Here's how the part is built. I have some questions about the finished solid (model axes, mm). A direction names the side the tool comes from. Coordinates: 2 decimals unless noted, no trailing zeros. Write each loop counter-clockwise with the first axis right and the second up, starting at its lowest first coordinate (ties: lowest second). Pieces come first, ordered by that corner, then holes.
```python
from build123d import *

# Parameters (mm, degrees)
EXTRUDE1_DEPTH      = 3
EXTRUDE1_DEPTH_BACK = 3
SKETCH2_OUTSIDE_W   = 52.392
SKETCH2_OUTSIDE_H   = 53.94
SKETCH2_OUTSIDE_R   = 5
CUT_EXTRUDE1_DEPTH  = 10.712534856
CUT_EXTRUDE1_DRAFT  = 60
SKETCH3_OUTSIDE_W   = 52.392
SKETCH3_OUTSIDE_H   = 53.94
SKETCH3_OUTSIDE_R   = 5
CUT_EXTRUDE2_DEPTH  = 10.712534856
CUT_EXTRUDE2_DRAFT  = 60
SKETCH4_R           = 3
CUT_EXTRUDE3_DEPTH  = 10.712534856
CUT_EXTRUDE7_DEPTH  = 0.635


with BuildPart() as part:
    # Sketch1 → Extrude1 (new, two sides: drawn at the far end of the back side and taken through both)
    with BuildSketch(Plane.XY.offset(-EXTRUDE1_DEPTH_BACK)):
        Polygon((0, 5.773502692), (-5, 2.886751346), (-5, -2.886751346), (0, -5.773502692), (5, -2.886751346), (5, 2.886751346), align=None)
    extrude(amount=EXTRUDE1_DEPTH + EXTRUDE1_DEPTH_BACK)


with BuildPart() as cut_extrude1_tool:
    # Sketch2 outside → Cut-Extrude1 (with draft: the straight prism first)
    with BuildSketch(Plane(origin=(0, 0, 3), x_dir=(-1, 0, 0), z_dir=(0, 0, -1))):
        Rectangle(SKETCH2_OUTSIDE_W, SKETCH2_OUTSIDE_H)
        Circle(SKETCH2_OUTSIDE_R, mode=Mode.SUBTRACT)
    extrude(amount=CUT_EXTRUDE1_DEPTH)
    # Cut-Extrude1: the draft: its side faces are tilted about the plane it starts from
    cut_extrude1_sides = [cut_extrude1_tool.faces().sort_by_distance(p)[0] for p in [
        (0, -26.97, -2.356267428),
        (-26.196, 0, -2.356267428),
        (0, 26.97, -2.356267428),
        (26.196, 0, -2.356267428),
        (5, 0, -2.356267428),
    ]]
    draft(cut_extrude1_sides, Plane(origin=(0, 0, 3), x_dir=(-1, 0, 0), z_dir=(0, 0, -1)), CUT_EXTRUDE1_DRAFT)


with BuildPart() as part_1:
    add(part.part)

    # Cut-Extrude1: cut by cut_extrude1_tool
    add(cut_extrude1_tool.part, mode=Mode.SUBTRACT)


with BuildPart() as cut_extrude2_tool:
    # Sketch3 outside → Cut-Extrude2 (with draft: the straight prism first)
    with BuildSketch(Plane.XY.offset(-3)):
        Rectangle(SKETCH3_OUTSIDE_W, SKETCH3_OUTSIDE_H)
        Circle(SKETCH3_OUTSIDE_R, mode=Mode.SUBTRACT)
    extrude(amount=CUT_EXTRUDE2_DEPTH)
    # Cut-Extrude2: the draft: its side faces are tilted about the plane it starts from
    cut_extrude2_sides = [cut_extrude2_tool.faces().sort_by_distance(p)[0] for p in [
        (0, -26.97, 2.356267428),
        (26.196, 0, 2.356267428),
        (0, 26.97, 2.356267428),
        (-26.196, 0, 2.356267428),
        (-5, 0, 2.356267428),
    ]]
    draft(cut_extrude2_sides, Plane.XY.offset(-3), CUT_EXTRUDE2_DRAFT)


with BuildPart() as part_2:
    add(part_1.part)

    # Cut-Extrude2: cut by cut_extrude2_tool
    add(cut_extrude2_tool.part, mode=Mode.SUBTRACT)

    # Sketch4 → Cut-Extrude3 (cut, through all)
    with BuildSketch(Plane(origin=(0, 0, -3), x_dir=(-1, 0, 0), z_dir=(0, 0, -1))):
        Circle(SKETCH4_R)
    extrude(amount=-CUT_EXTRUDE3_DEPTH, mode=Mode.SUBTRACT)

    # Sketch12 → Cut-Extrude7 (cut)
    with BuildSketch(Plane.XY.offset(3)):
        Polygon((-3.1, 0), (-5, 1.096965511), (-5, -1.096965511), align=None)
        Polygon((3.1, 0), (5, -1.096965511), (5, 1.096965511), align=None)
    extrude(amount=-CUT_EXTRUDE7_DEPTH, mode=Mode.SUBTRACT)


solid = part_2.part
```
1) I need wall thicknesses on probe 1 along X at (y, z) = (1.5, -1.35); probe 2 along Y at (x, z) = (2.75, -1.7); probe 3 along Y at (x, z) = (2, -0.75). Which ranges of each line are inside material? Lowest first, please.
Values follow:
probe 1: x = -5 to -2.6, 2.6 to 5
probe 2: y = -4.19 to -1.2, 1.2 to 4.19
probe 3: y = -4.62 to -2.24, 2.24 to 4.62
2) We'd pull the mould along X, two halves only. Please class faces 1 (the face through (3, 0, 0)), 2 (the face through (0.013, -5.184, 2.894)), 3 (the face through (4.063, 0.556, 2.687)): pulls with the +X half, pulls with the -X half, needs draft (parallel to the pull), parting line crosses it, or undercut.
Values follow:
face 1: undercut
face 2: parting line crosses it
face 3: pulls with the +X half
3) Will these pins go through, and if not, where does the flat tip stop? pin 1 (3 mm diameter, centred on x = 3.5, z = 2.5, fed in from +Y); pin 2 (5.5 mm diameter, centred on x = 0, y = 0, fed in from -Z); pin 3 (1 mm diameter, centred on x = -1, z = -1.5, fed in from +Y).
Values follow:
pin 1: stops at y = 4.62
pin 2: passes through
pin 3: stops at y = 5.48
4) On a 3-axis mill with a long thin cutter (end or side, diameter ignored), from which of +Z, -Z, +X, -X, +Y, -Y can I reach the whole of each face in a straight line? I mean faces 4 (the face through (-4.037, 0.541, 2.687)), 5 (the face through (-0.013, 5.184, 2.894)), 6 (the face through (4.037, -0.541, 2.687)). Say none if no direction works.
Values follow:
face 4: +Z, -X
face 5: +Z, +Y
face 6: +Z, +X
5) Imagine slicing it at A-A on z = -1.3. Please give me the cut outline in (x, y).
Values follow:
outline: (-5, -2.89) - (0, -5.77) - (5, -2.89) - (5, 2.89) - (0, 5.77) - (-5, 2.89) - close; hole circle Ø6 at (0, 0)
